from build123d import *

# Parameters (mm, degrees)
SKETCH_R           = 2
PAD_DEPTH          = 18
POCKET_DEPTH       = 8.25
POCKET007002_DEPTH = 27.001
SKETCH003_R        = 2.35
POCKET007003_DEPTH = 6
SKETCH004_R        = 2.35
POCKET007004_DEPTH = 7
SKETCH005_R        = 2.75
POCKET007005_DEPTH = 0.75
SKETCH006_R        = 2.75
POCKET007006_DEPTH = 0.75
CHAMFER_SIZE       = 1
CHAMFER001_SIZE    = 2


with BuildPart() as part:
    # Sketch → Pad (new body)
    with BuildSketch(Plane.YZ):
        Polygon((2.125, 0), (2.125, -8.25), (5.625, -8.25), (5.625, -16.5), (2.125, -16.5), (2.125, -27), (13.125, -27), (13.125, -16.5), (10.625, -16.5), (10.625, -8.25), (13.125, -8.25), (13.125, 0), align=None)
        with Locations((9.125, -22)):
            Circle(SKETCH_R, mode=Mode.SUBTRACT)
    extrude(amount=PAD_DEPTH)

    # Sketch001 (on Face10 of Pad) → Pocket (cut)
    with BuildSketch(Plane.YX.offset(8.25)):
        with BuildLine():
            Line((2.125, 18), (7.5, 18))
            Line((7.5, 18), (7.5, 13))
            Line((7.5, 13), (10, 13))
            Line((10, 13), (10, 18))
            Line((10, 18), (10.625, 18))
            Line((10.625, 18), (10.625, 10))
            Line((10.625, 10), (7.625, 10))
            Line((7.625, 10), (5.6200366733, 3.7653591075))
            ThreePointArc((5.6200366733, 3.7653591075), (7.4780711036, 0.5550889122), (10.4850277531, 2.7268021481))
            Line((10.4850277531, 2.7268021481), (10.625, 4))
            Line((10.625, 4), (10.625, 0))
            Line((10.625, 0), (2.125, 0))
            Line((2.125, 0), (2.125, 18))
        make_face()
    extrude(amount=POCKET_DEPTH, mode=Mode.SUBTRACT)

    # Sketch002 (on Face8 of Pocket) → Pocket007002 (cut, through all)
    with BuildSketch(Plane.YX.offset(27)):
        Polygon((2.125, 18), (4.125, 18), (4.125, 13), (2.125, 6.5), align=None)
    extrude(amount=-POCKET007002_DEPTH, mode=Mode.SUBTRACT)

    # Sketch003 (on Face23 of Pocket007002) → Pocket007003 (cut)
    with BuildSketch(Plane(origin=(-0.0351351351, 0.1141891892, 0), x_dir=(0, 0, -1), z_dir=(0.2940858488, -0.9557790087, 0))):
        with Locations((4.25, 10.375)):
            Circle(SKETCH003_R)
        with Locations((21.5, 10.375)):
            Circle(SKETCH003_R)
    extrude(amount=-POCKET007003_DEPTH, mode=Mode.SUBTRACT)

    # Sketch004 (on Face5 of Pocket007003) → Pocket007004 (cut)
    with BuildSketch(Plane(origin=(0, 0, 0), x_dir=(0, -1, 0), z_dir=(0, 0, 1))):
        with Locations((-8, 3.5)):
            Circle(SKETCH004_R)
    extrude(amount=-POCKET007004_DEPTH, mode=Mode.SUBTRACT)

    # Sketch005 (on Face5 of Pocket007004) → Pocket007005 (cut)
    with BuildSketch(Plane(origin=(0, 0, 0), x_dir=(0, -1, 0), z_dir=(0, 0, 1))):
        with Locations((-8, 3.5)):
            Circle(SKETCH005_R)
    extrude(amount=-POCKET007005_DEPTH, mode=Mode.SUBTRACT)

    # Sketch006 (on Face4 of Pocket007005) → Pocket007006 (cut)
    with BuildSketch(Plane(origin=(-0.0351351351, 0.1141891892, 0), x_dir=(0, 0, -1), z_dir=(0.2940858488, -0.9557790087, 0))):
        with Locations((21.5, 10.375)):
            Circle(SKETCH006_R)
        with Locations((4.25, 10.375)):
            Circle(SKETCH006_R)
    extrude(amount=-POCKET007006_DEPTH, mode=Mode.SUBTRACT)

    # Chamfer
    chamfer_edges = [part.edges().sort_by_distance(p)[0] for p in [
        (3.25, 2.125, -16.5),
        (3.25, 2.125, -8.25),
        (15.5, 4.125, -8.25),
        (15.5, 4.125, -16.5),
    ]]
    chamfer(chamfer_edges, length=CHAMFER_SIZE)

    # Chamfer001
    chamfer001_edges = [part.edges().sort_by_distance(p)[0] for p in [
        (9, 13.125, -16.5),
        (9, 13.125, -8.25),
    ]]
    chamfer(chamfer001_edges, length=CHAMFER001_SIZE)


solid = part.part
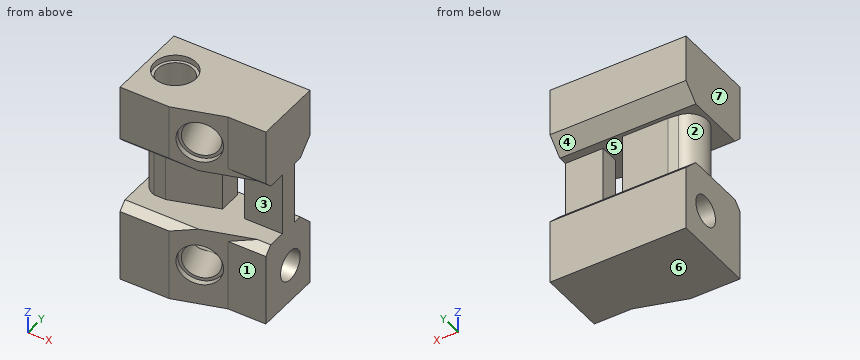
Input: part model. Units: mm. Frame: model coordinates. Face numbers are marked on the shaded views. A direction names the side the tool comes from. Coordinates: 2 decimals unless noted, no trailing zeros. Order: outer loops, then holes, each group sorted by start corner. A loop starts at its lowest first (then second) coordinate and runs counter-clockwise, first axis right, second up. Notation, with made-up numbers: M -16.5,32 L 25.5,32 A23 ccw 25.5,40 Z; hole C 55.25,-35 d8. An arc over 180 degrees is marked long. Answer in a Markdown table with one row per item.
(1) Access query for the marked faces 1, 2, 3 and 4. Directions: +Z, -Z, +X, -X, +Y, -Y. A direction counts if a zero-diameter tool reaches every point of the face in a straight line with its end or side. Return the directions, or none.
Numbers:
| item | result |
|---|---|
| face 1 | +Z, -Z, +X, -Y |
| face 2 | -X |
| face 3 | +X, -Y |
| face 4 | +X, -X, +Y |
(2) Section query C-C, the plane x = 3.5. Output: boundary loops of the cut face in (y, z) (3 decimals).
Numbers:
| item | result |
|---|---|
| outline | M 2.125,-27 L 13.125,-27 L 13.125,-18.5 L 11.125,-16.5 L 10.57,-16.5 L 10.57,-8.25 L 11.125,-8.25 L 13.125,-6.25 L 13.125,0 L 10.75,0 L 10.75,-0.75 L 10.35,-0.75 L 10.35,-7 L 5.65,-7 L 5.65,-0.75 L 5.25,-0.75 L 5.25,0 L 2.125,0 L 2.125,-7.25 L 3.125,-8.25 L 5.625,-8.25 L 5.625,-16.5 L 3.125,-16.5 L 2.125,-17.5 Z; hole C 9.125,-22 d4 |
(3) Section query A-A, the plane z = -13. Output: boundary loops of the cut face in (x, y) (3 decimals).
Numbers:
| item | result |
|---|---|
| outline | M 2.219,5.625 L 3.781,5.625 L 10,7.625 L 10,10.625 L 4,10.625 L 2.727,10.485 A2.5 ccw Z; M 13,7.5 L 18,7.5 L 18,10 L 13,10 Z |
(4) Draft query along Z for the marked faces 5, 6 and 7. Return one class per face: pulls with the +Z half, pulls with the -Z half, needs draft (parallel to the pull), parting line crosses it, or undercut.
Numbers:
| item | result |
|---|---|
| face 5 | undercut |
| face 6 | pulls with the -Z half |
| face 7 | needs draft |
(5) Section query D-D, the plane z = -4. Output: boundary loops of the cut face in (x, y) (3 decimals).
Numbers:
| item | result |
|---|---|
| outline | M 0,2.125 L 6.5,2.125 L 7.264,2.36 L 7.043,3.077 L 7.427,3.195 L 5.883,8.213 L 10.35,9.587 L 11.894,4.569 L 12.278,4.688 L 12.499,3.971 L 13,4.125 L 18,4.125 L 18,13.125 L 0,13.125 Z; hole C 3.5,8 d4.7 |
(6) Contact query for flat-ended pins moving along their axis: pin 1 Ø4 at (x, y) = (3.5, 8) entering from +Z; pin 2 Ø1.5 at (x, z) = (15, -21.5) entering from -Y (3 decimals); pin 3 Ø1 at (y, z) = (10.5, -14.5) entering from -X. Output: stop coordinate, or through.
Numbers:
| item | result |
|---|---|
| pin 1 | stops at z = -7 |
| pin 2 | stops at y = 4.125 |
| pin 3 | stops at x = 1.5 |
(7) Section query B-B, the plane z = -20.5. Output: boundary loops of the cut face in (x, y) (3 decimals), plus the area to 3 significant figures.
Numbers:
| item | result |
|---|---|
| outline | M 0,2.125 L 6.5,2.125 L 7.433,2.412 L 7.212,3.129 L 7.628,3.257 L 6.229,7.802 L 0,7.802 Z; M 0,10.448 L 18,10.448 L 18,13.125 L 0,13.125 Z; M 10.679,7.802 L 11.693,4.508 L 12.109,4.636 L 12.33,3.919 L 13,4.125 L 18,4.125 L 18,7.802 Z |
| area | 113 mm^2 |
(8) Material intervals for line 1 (X direction, y = 8, z = -0.3); line 2 (Z direction, x = 17.25, y = 5.75); line 3 (Z direction, x = 9.5, y = 6.25), sorted ascending. Write a range as [from, to].
Numbers:
| item | result |
|---|---|
| line 1 | x = [0, 0.75], [6.25, 18] |
| line 2 | z = [-27, -16.5], [-8.25, 0] |
| line 3 | z = [-27, -23.79], [-19.21, -16.5], [-8.25, -6.54], [-1.96, 0] |
